from build123d import *

# Parameters (mm, degrees)
SKETCH1_W           = 42
SKETCH1_H           = 42
BOSS_EXTRUDE1_DEPTH = 47
SKETCH2_R           = 2.5
BOSS_EXTRUDE4_DEPTH = 24
SKETCH2_5_R         = 11
SKETCH2_5_R_2       = 2.5
BOSS_EXTRUDE5_DEPTH = 2
CIRPATTERN1_COUNT   = 4
FILLET1_R           = 5
SKETCH14_W          = 5.6
SKETCH14_H          = 15
BOSS_EXTRUDE6_DEPTH = 6


with BuildPart() as part:
    # Sketch1 → Boss-Extrude1 (new body)
    with BuildSketch(Plane.XY):
        Rectangle(SKETCH1_W, SKETCH1_H)
    extrude(amount=BOSS_EXTRUDE1_DEPTH)

    # Sketch2 → Boss-Extrude4 (add)
    with BuildSketch(Plane.XY.offset(47)):
        Circle(SKETCH2_R)
    extrude(amount=BOSS_EXTRUDE4_DEPTH)

    # Sketch2_5 → Boss-Extrude5 (add)
    with BuildSketch(Plane.XY.offset(47)):
        Circle(SKETCH2_5_R)
        Circle(SKETCH2_5_R_2, mode=Mode.SUBTRACT)
    extrude(amount=BOSS_EXTRUDE5_DEPTH)

    # Sketch12 → M3 Tapped Hole3 (revolve, cut)
    with BuildSketch(Plane(origin=(-15.5, 15.5, 47), x_dir=(0, -1, 0), z_dir=(1, 0, 0))):
        Polygon((0, 0), (0, 6.751075774), (1.25, 6), (1.25, 0), align=None)
    m3_tapped_hole3 = revolve(axis=Axis((-15.5, 15.5, 53.35), (0, 0, -1)), mode=Mode.SUBTRACT)

    # CirPattern1: M3 Tapped Hole3 ×4 about axis
    cirpattern1_axis = Axis((0, 0, 0), (0, 0, 1))
    for i in range(1, CIRPATTERN1_COUNT):
        add(m3_tapped_hole3.rotate(cirpattern1_axis, i * 360 / CIRPATTERN1_COUNT), mode=Mode.SUBTRACT)

    # Fillet1
    fillet1_edges = [part.edges().sort_by_distance(p)[0] for p in [
        (-21, -21, 23.5),
        (-21, 21, 23.5),
        (21, 21, 23.5),
        (21, -21, 23.5),
    ]]
    fillet(fillet1_edges, radius=FILLET1_R)

    # Sketch14 → Boss-Extrude6 (add)
    with BuildSketch(Plane(origin=(21, 0, 0), x_dir=(0, 0, -1), z_dir=(1, 0, 0))):
        with Locations((-7.2, 0)):
            Rectangle(SKETCH14_W, SKETCH14_H)
    extrude(amount=BOSS_EXTRUDE6_DEPTH)


solid = part.part
Source: CAD feature listing. Evaluate the final solid. Frame: model axes, mm. A direction names the side the tool comes from. Give positions to 0.01 mm unless a question says otherwise; leave off trailing zeros. Write each loop counter-clockwise with the first axis right and the second up, starting at its lowest first coordinate (ties: lowest second). Pieces come first, ordered by that corner, then holes. Notation, with made-up numbers: (-37.75, 51) -> (-6.75, 51) arc R31 ccw to (-6.75, 90) -> close; hole circle Ø1 at (-14, -15.75). An arc over 180 degrees is marked (long way). Return JSON: item names as keys, results as strings. Group by question number.
1. Section D-D, the plane z = 24. Output: boundary loops of the cut face in (x, y).
2. Mould query, pull axis X, two halves, no side actions, for faces 1 (the face through (-15.55, -15.29, 40.38)), 2 (the face through (0, 0, 0)), 3 (the face through (-21, 0, 23)). Classes: +X half, -X half, draft (parallel to the pull), parting line (faces both ways), or undercut.
3. Pin query (flat end, axial travel): pin 1 Ø4 at (x, y) = (4, -1) entering from +Z; pin 2 Ø2 at (x, y) = (15.5, 15.5) entering from +Z; pin 3 Ø1.8 at (x, y) = (24, -2.5) entering from -Z; pin 4 Ø3 at (x, y) = (23, -3.5) entering from +Z. Return the tip coordinate at first contact, or that it passes through.
4. Section A-A, the plane z = 5.5. Output: boundary loops of the cut face in (x, y), then the cut area to 3 significant figures.
5. Section B-B, the plane y = 0. Output: boundary loops of the cut face in (x, z), then the cut area to 3 significant figures.
6. Section C-C, the plane x = 0. Output: boundary loops of the cut face in (y, z).
7. Access query for faces 4 (the face through (24, 7.5, 7)), 5 (the face through (-16.345, 16.421, 44.042)), 6 (the face through (24, 0, 4.4)). Directions: +Z, -Z, +X, -X, +Y, -Y. A direction counts if a zero-diameter tool reaches every point of the face in a straight line with its end or side. Return the directions, or none.
8. Material intervals for line 1 (X direction, y = 15, z = 45); line 2 (Z direction, x = 2.5, y = -9); line 3 (Z direction, x = 14, y = 18), sorted ascending. Write a range as from..to.
Determined:
{
 "1": {"outline": "(-21, -16) arc R5 ccw to (-16, -21) -> (16, -21) arc R5 ccw to (21, -16) -> (21, 16) arc R5 ccw to (16, 21) -> (-16, 21) arc R5 ccw to (-21, 16) -> close"},
 "2": {"face 1": "undercut", "face 2": "draft", "face 3": "-X half"},
 "3": {"pin 1": "stops at z = 71", "pin 2": "stops at z = 40.85", "pin 3": "stops at z = 4.4", "pin 4": "stops at z = 10"},
 "4": {"outline": "(-21, -16) arc R5 ccw to (-16, -21) -> (16, -21) arc R5 ccw to (21, -16) -> (21, -7.5) -> (27, -7.5) -> (27, 7.5) -> (21, 7.5) -> (21, 16) arc R5 ccw to (16, 21) -> (-16, 21) arc R5 ccw to (-21, 16) -> close", "area": "1,830 mm2"},
 "5": {"outline": "(-21, 0) -> (21, 0) -> (21, 4.4) -> (27, 4.4) -> (27, 10) -> (21, 10) -> (21, 47) -> (11, 47) -> (11, 49) -> (2.5, 49) -> (2.5, 71) -> (-2.5, 71) -> (-2.5, 49) -> (-11, 49) -> (-11, 47) -> (-21, 47) -> close", "area": "2,160 mm2"},
 "6": {"outline": "(-21, 0) -> (21, 0) -> (21, 47) -> (11, 47) -> (11, 49) -> (2.5, 49) -> (2.5, 71) -> (-2.5, 71) -> (-2.5, 49) -> (-11, 49) -> (-11, 47) -> (-21, 47) -> close"},
 "7": {"face 4": "+Z, -Z, +X, +Y", "face 5": "+Z", "face 6": "-Z, +X, +Y, -Y"},
 "8": {"line 1": "x = -21..-16.65, -14.35..14.35, 16.65..21", "line 2": "z = 0..49", "line 3": "z = 0..47"}
}
